For this review, take the finished solid that the model builds, in its own axes (mm). A direction names the side the tool comes from. Round coordinates to 2 decimals unless told otherwise and drop trailing zeros. Order: outer loops, then holes, each group sorted by start corner. A loop starts at its lowest first (then second) coordinate and runs counter-clockwise, first axis right, second up. Notation, with made-up numbers: (68, 24) -> (86, 24) arc R26 cw to (86, 40) -> close; hole circle Ø5 at (35.25, -39.75). An arc over 180 degrees is marked (long way). Use a Markdown table: item, result. Add a question column.
1) Consider section D-D (z = 38). State the section outline as (x, y) points.
2) Consider section B-B (z = 17). State the section outline as (x, y) points.
3) Machinability: for faces 5 (the face through (52.507, -14.67, 30.21)), 6 (the face through (20, -73, 30)), 7 (the face through (10, -72, 35)), 8 (the face through (49, -50, 13)), which of the approach directions +Z, -Z, +X, -X, +Y, -Y give a long, thin tool a straight path to every point of the face, cutting with its end or side? Answer none if there is none.
4) Wall thickness on line 1 along Y through (x, z) = (60, 24.5); line 2 along Z through (x, y) = (63, -64); line 3 along X through (y, z) = (-16, 38.5): over which ranges is each line inside the solid? List them lowest first. Write a range as [from, to].
5) Draft analysis for pull direction Y (two halves, no side actions). For faces 1 (the face through (0, -41, 17)), 2 (the face through (49, 0, 23)), 3 (the face through (10, -65, 30)), 4 (the face through (49, -80, 17)), state which applies: pulls with the +Y half, pulls with the -Y half, needs draft (parallel to the pull), parting line crosses it, or undercut.
6) Consider section C-C (x = 60). State the section outline as (y, z) points, plus the area to 3 significant figures.
7) Clearance check with flat-ended pins moving along their axes: P1, Ø3, axis at x = 11.5, z = 28, coming from the +Y side; P2, Ø12, axis at x = 60, y = -15, coming from the +Z side; P3, Ø2, axis at x = 50.5, y = -57, coming from the +Z side; P4, Ø12, axis at x = 13.5, y = -76, coming from the +Z side. State where each tip first meets the part, or that it passes through.
8) Consider section A-A (y = -31). State the section outline as (x, z) points, plus the area to 3 significant figures.
```python
from build123d import *

# Parameters (mm, degrees)
F0_W      = 100
F0_H      = 45
F1_DEPTH  = 80
F2_R      = 7.5
F3_DEPTH  = 30
F4_R      = 70
F5_DEPTH  = 20
F6_W      = 20
F6_H      = 15
F7_DEPTH  = 10
F10_DEPTH = 25.001
F12_DEPTH = 80.001


with BuildPart() as f1:
    # F0 (on Front) → F1 (new body)
    with BuildSketch(Plane.XZ):
        with Locations((50, 22.5)):
            Rectangle(F0_W, F0_H)
    extrude(amount=F1_DEPTH)

    # F2 (on face) → F3 (cut)
    with BuildSketch(Plane.XY.offset(45)):
        with Locations((60, -15)):
            Circle(F2_R)
    extrude(amount=-F3_DEPTH, mode=Mode.SUBTRACT)

    # F4 (on face) → F5 (cut)
    with BuildSketch(Plane.XY.offset(45)):
        with Locations((0, -80)):
            Circle(F4_R)
    extrude(amount=-F5_DEPTH, mode=Mode.SUBTRACT)

    # F6 (on face) → F7 (join)
    with BuildSketch(Plane.XY.offset(25)):
        with Locations((10, -72.5)):
            Rectangle(F6_W, F6_H)
    extrude(amount=F7_DEPTH)

    # F9 (on face) → F10 (cut, through all)
    with BuildSketch(Plane.XY.offset(25)):
        with BuildLine():
            ThreePointArc((63.2455532034, -50), (51.4535762322, -32.5391793906), (35, -19.3782217351))
            Line((35, -19.3782217351), (35, -50))
            Line((35, -50), (63.2455532034, -50))
        make_face()
    extrude(amount=-F10_DEPTH, mode=Mode.SUBTRACT)

    # F11 (on face) → F12 (cut, through all)
    with BuildSketch(Plane.XZ.offset(80)):
        with BuildLine():
            ThreePointArc((83.6190264738, 45), (95.7773967757, 23.944395449), (100, 0))
            Line((100, 0), (100, 45))
            Line((100, 45), (83.6190264738, 45))
        make_face()
    extrude(amount=-F12_DEPTH, mode=Mode.SUBTRACT)


solid = f1.part
```
Results list:
| question | item | result |
|---|---|---|
| 1 | outline | (0, -10) arc R70 cw to (70, -80) -> (88.79, -80) -> (88.79, 0) -> (0, 0) -> close; hole circle Ø15 at (60, -15) |
| 2 | outline | (0, -80) -> (97.9, -80) -> (97.9, 0) -> (0, 0) -> close; hole (35, -50) -> (63.25, -50) arc R70 ccw to (35, -19.38) -> close; hole circle Ø15 at (60, -15) |
| 3 | face 5 | +Z |
| 3 | face 6 | +Z, -Y |
| 3 | face 7 | +Z, -X, -Y |
| 3 | face 8 | +Z, -Z |
| 4 | line 1 | [-80, -50], [-43.94, -22.5], [-7.5, 0] |
| 4 | line 2 | [0, 25] |
| 4 | line 3 | [28.35, 52.57], [67.43, 88.46] |
| 5 | face 1 | needs draft |
| 5 | face 2 | pulls with the +Y half |
| 5 | face 3 | undercut |
| 5 | face 4 | pulls with the -Y half |
| 6 | outline | (-80, 0) -> (-50, 0) -> (-50, 25) -> (-80, 25) -> close; (-43.94, 0) -> (0, 0) -> (0, 45) -> (-7.5, 45) -> (-7.5, 15) -> (-22.5, 15) -> (-22.5, 45) -> (-43.94, 45) -> close |
| 6 | area | 2,280 mm2 |
| 7 | P1 | y = 0 |
| 7 | P2 | z = 15 |
| 7 | P3 | z = 25 |
| 7 | P4 | z = 35 |
| 8 | outline | (0, 0) -> (35, 0) -> (35, 25) -> (0, 25) -> close; (49.99, 0) -> (100, 0) arc R70 ccw to (83.62, 45) -> (49.99, 45) -> close |
| 8 | area | 2,890 mm2 |
